Could you check a few things on this model? Use its own coordinates, in mm. Face numbers are marked on the shaded views. A direction names the side the tool comes from. Round coordinates to 2 decimals unless told otherwise and drop trailing zeros. Write each loop counter-clockwise with the first axis right and the second up, starting at its lowest first coordinate (ties: lowest second). Pieces come first, ordered by that corner, then holes. Notation, with made-up numbers: M 14.5,61 L 61.5,61 A24 cw 61.5,99 Z; hole C -28,34.5 d10. An arc over 180 degrees is marked long. One line per item, written item: value. Start each with the question number.
(1) Which directions (+Z, -Z, +X, -X, +Y, -Y) give clear straight access to the entire face, cutting with the end or side of a thin tool? Please do the marked faces 1, 2, 3, 4 and 5.
(2) I want a section at C-C on y = 114. Please give me the cut outline in (x, z), and give its area (3 significant figures).
(3) I want a section at D-D on z = 25. Please give me the cut outline in (x, y).
(4) I'm going to push flat-ended pins straight in: pin 1 Ø4.5 at (x, z) = (-73.15, 20) entering from -Y; pin 2 Ø0.8 at (y, z) = (18.5, 0.5) entering from +X; pin 3 Ø0.6 at (y, z) = (1, 38.5) entering from +X. Where does each tip first touch, or does it pass through?
(5) I want a section at B-B on z = 12. Please give me the cut outline in (x, y).
(6) I want a section at A-A on x = 0. Please give me the cut outline in (y, z).
(7) If I drill on L1, parallel to X at y = 38.5, z = 25; L2, parallel to Y at x = -77.5, z = 30.5; L3, parallel to X at y = 91, z = 19, over which ranges is the centre line in solid material (lowest first)?
(8) Thinking about a two-plate mould opening in X: for the marked faces 6, 7, 8 and 9, which applies, released by +X, released by -X, zero draft, split by the parting line, or undercut?
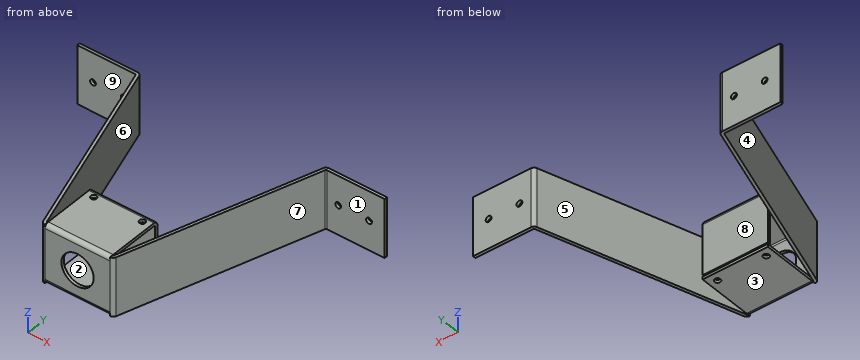
```python
from build123d import *

# Parameters (mm, degrees)
BASE_FLANGE1_DEPTH           = 40
EDGE_FLANGE1_STRIP_W         = 9.4732
EDGE_FLANGE1_STRIP_H         = 2
EDGE_FLANGE1_STRIP_CUT_DEPTH = 44.47497737
EDGE_FLANGE1_DEPTH           = 44.47497737
EDGE_FLANGE2_STRIP_W         = 9.4732
EDGE_FLANGE2_STRIP_H         = 2
EDGE_FLANGE2_STRIP_CUT_DEPTH = 44.47497737
EDGE_FLANGE2_DEPTH           = 44.47497737
EDGE_FLANGE3_STRIP_W         = 9.4732
EDGE_FLANGE3_STRIP_H         = 2
EDGE_FLANGE3_STRIP_CUT_DEPTH = 44.47497737
EDGE_FLANGE3_DEPTH           = 44.47497737
CUT_EXTRUDE1_REACH           = 175.247
SKETCH28_R                   = 11
SKETCH28_R_2                 = 2
SKETCH29_R                   = 2
CUT_EXTRUDE2_DEPTH           = 174.246707232


# Sheet-metal steps are written as plain solids
with BuildPart() as part:
    # Sketch1 → Base-Flange1 (new body)
    with BuildSketch(Plane.XY):
        with BuildLine():
            Line((104.835211483, 130), (65.376911342, 130))
            ThreePointArc((65.376911342, 130), (64.940513549, 129.856810925), (64.67378015, 129.482913293))
            Line((64.67378015, 129.482913293), (24.849746113, 1.921069076))
            ThreePointArc((24.849746113, 1.921069076), (23.858784098, 0.531972879), (22.237488685, 0))
            Line((22.237488685, 0), (-22.237488685, 0))
            ThreePointArc((-22.237488685, 0), (-23.858784098, 0.531972879), (-24.849746113, 1.921069076))
            Line((-24.849746113, 1.921069076), (-64.67378015, 129.482913293))
            ThreePointArc((-64.67378015, 129.482913293), (-64.940513549, 129.856810925), (-65.376911342, 130))
            Line((-65.376911342, 130), (-104.835211483, 130))
            Line((-104.835211483, 130), (-104.835211483, 132))
            Line((-104.835211483, 132), (-65.376911342, 132))
            ThreePointArc((-65.376911342, 132), (-63.755615929, 131.468027121), (-62.764653914, 130.078930924))
            Line((-62.764653914, 130.078930924), (-22.940619877, 2.517086707))
            ThreePointArc((-22.940619877, 2.517086707), (-22.673886478, 2.143189075), (-22.237488685, 2))
            Line((-22.237488685, 2), (22.237488685, 2))
            ThreePointArc((22.237488685, 2), (22.673886478, 2.143189075), (22.940619877, 2.517086707))
            Line((22.940619877, 2.517086707), (62.764653914, 130.078930924))
            ThreePointArc((62.764653914, 130.078930924), (63.755615929, 131.468027121), (65.376911342, 132))
            Line((65.376911342, 132), (104.835211483, 132))
            Line((104.835211483, 132), (104.835211483, 130))
        make_face()
    extrude(amount=BASE_FLANGE1_DEPTH)

    # Edge-Flange1 strip (across the edge) → Edge-Flange1 strip cut (cut)
    with BuildSketch(Plane(origin=(22.237488685, 2, 0), x_dir=(0, 0, 1), z_dir=(-1, 0, 0))):
        with Locations((-2, -1)):
            Rectangle(EDGE_FLANGE1_STRIP_W, EDGE_FLANGE1_STRIP_H)
    extrude(amount=EDGE_FLANGE1_STRIP_CUT_DEPTH, mode=Mode.SUBTRACT)

    # Edge-Flange1 section (across the edge) → Edge-Flange1 (add)
    with BuildSketch(Plane(origin=(22.237488685, 2, 0), x_dir=(0, 0, 1), z_dir=(-1, 0, 0))):
        with BuildLine():
            Line((0, 0.7366), (0, 38))
            Line((0, 38), (2, 38))
            Line((2, 38), (2, 0.7366))
            ThreePointArc((2, 0.7366), (2.215745145, 0.215745145), (2.7366, 0))
            Line((2.7366, 0), (2.7366, -2))
            ThreePointArc((2.7366, -2), (0.801531583, -1.198468417), (0, 0.7366))
        make_face()
    extrude(amount=EDGE_FLANGE1_DEPTH)

    # Edge-Flange2 strip (across the edge) → Edge-Flange2 strip cut (cut)
    with BuildSketch(Plane(origin=(-22.237488685, 2, 40), x_dir=(0, 0, -1), z_dir=(1, 0, 0))):
        with Locations((-2, -1)):
            Rectangle(EDGE_FLANGE2_STRIP_W, EDGE_FLANGE2_STRIP_H)
    extrude(amount=EDGE_FLANGE2_STRIP_CUT_DEPTH, mode=Mode.SUBTRACT)

    # Edge-Flange2 section (across the edge) → Edge-Flange2 (add)
    with BuildSketch(Plane(origin=(-22.237488685, 2, 40), x_dir=(0, 0, -1), z_dir=(1, 0, 0))):
        with BuildLine():
            Line((0, 0.7366), (0, 38))
            Line((0, 38), (2, 38))
            Line((2, 38), (2, 0.7366))
            ThreePointArc((2, 0.7366), (2.215745145, 0.215745145), (2.7366, 0))
            Line((2.7366, 0), (2.7366, -2))
            ThreePointArc((2.7366, -2), (0.801531583, -1.198468417), (0, 0.7366))
        make_face()
    extrude(amount=EDGE_FLANGE2_DEPTH)

    # Edge-Flange3 strip (across the edge) → Edge-Flange3 strip cut (cut)
    with BuildSketch(Plane(origin=(-22.237488685, 40, 38), x_dir=(0, -1, 0), z_dir=(1, 0, 0))):
        with Locations((-2, -1)):
            Rectangle(EDGE_FLANGE3_STRIP_W, EDGE_FLANGE3_STRIP_H)
    extrude(amount=EDGE_FLANGE3_STRIP_CUT_DEPTH, mode=Mode.SUBTRACT)

    # Edge-Flange3 section (across the edge) → Edge-Flange3 (add)
    with BuildSketch(Plane(origin=(-22.237488685, 40, 38), x_dir=(0, -1, 0), z_dir=(1, 0, 0))):
        with BuildLine():
            Line((0, 0.7366), (0, 35))
            Line((0, 35), (2, 35))
            Line((2, 35), (2, 0.7366))
            ThreePointArc((2, 0.7366), (2.215745145, 0.215745145), (2.7366, 0))
            Line((2.7366, 0), (2.7366, -2))
            ThreePointArc((2.7366, -2), (0.801531583, -1.198468417), (0, 0.7366))
        make_face()
    extrude(amount=EDGE_FLANGE3_DEPTH)

    # Sketch28 → Cut-Extrude1 (cut, up to next)
    with BuildSketch(Plane.XZ, mode=Mode.PRIVATE) as cut_extrude1_sk1:
        with Locations(Location((0, 20, 0), (0, 0, 270))):
            Circle(SKETCH28_R)
    cut_extrude1_tool1 = extrude(cut_extrude1_sk1.sketch, amount=-CUT_EXTRUDE1_REACH, mode=Mode.PRIVATE) & part.part
    # Sketch28 → Cut-Extrude1 (cut, up to next)
    with BuildSketch(Plane.XZ, mode=Mode.PRIVATE) as cut_extrude1_sk2:
        with Locations((73.154329826, 20)):
            Circle(SKETCH28_R_2)
    cut_extrude1_tool2 = extrude(cut_extrude1_sk2.sketch, amount=-CUT_EXTRUDE1_REACH, mode=Mode.PRIVATE) & part.part
    # Sketch28 → Cut-Extrude1 (cut, up to next)
    with BuildSketch(Plane.XZ, mode=Mode.PRIVATE) as cut_extrude1_sk3:
        with Locations((94.167570852, 20)):
            Circle(SKETCH28_R_2)
    cut_extrude1_tool3 = extrude(cut_extrude1_sk3.sketch, amount=-CUT_EXTRUDE1_REACH, mode=Mode.PRIVATE) & part.part
    # Sketch28 → Cut-Extrude1 (cut, up to next)
    with BuildSketch(Plane.XZ, mode=Mode.PRIVATE) as cut_extrude1_sk4:
        with Locations((-94.167570852, 20)):
            Circle(SKETCH28_R_2)
    cut_extrude1_tool4 = extrude(cut_extrude1_sk4.sketch, amount=-CUT_EXTRUDE1_REACH, mode=Mode.PRIVATE) & part.part
    # Sketch28 → Cut-Extrude1 (cut, up to next)
    with BuildSketch(Plane.XZ, mode=Mode.PRIVATE) as cut_extrude1_sk5:
        with Locations((-73.154329826, 20)):
            Circle(SKETCH28_R_2)
    cut_extrude1_tool5 = extrude(cut_extrude1_sk5.sketch, amount=-CUT_EXTRUDE1_REACH, mode=Mode.PRIVATE) & part.part
    add(cut_extrude1_tool1.solids().sort_by_distance((0, 0, 20))[0], mode=Mode.SUBTRACT)
    add(cut_extrude1_tool2.solids().sort_by_distance((73.15433, 0, 20))[0], mode=Mode.SUBTRACT)
    add(cut_extrude1_tool3.solids().sort_by_distance((94.167571, 0, 20))[0], mode=Mode.SUBTRACT)
    add(cut_extrude1_tool4.solids().sort_by_distance((-94.167571, 0, 20))[0], mode=Mode.SUBTRACT)
    add(cut_extrude1_tool5.solids().sort_by_distance((-73.15433, 0, 20))[0], mode=Mode.SUBTRACT)

    # Sketch29 → Cut-Extrude2 (cut, through all)
    with BuildSketch(Plane(origin=(0, 0, 0), x_dir=(-1, 0, 0), z_dir=(0, 0, -1))):
        with Locations(Location((-16.618744342, 34.381255658, 0), (0, 0, 90))):
            Circle(SKETCH29_R)
        with Locations(Location((16.618744342, 34.381255658, 0), (0, 0, 90))):
            Circle(SKETCH29_R)
    extrude(amount=-CUT_EXTRUDE2_DEPTH, mode=Mode.SUBTRACT)


solid = part.part
```
Found:
1. face 1: +Z, -Z, +X, -Y
1. face 2: +Y
1. face 3: -Z, +X, -X, +Y, -Y
1. face 4: +Z, -Z, -X, -Y
1. face 5: +Z, -Z, +Y
2. outline: M -59.84,0 L -57.74,0 L -57.74,40 L -59.84,40 Z; M 57.74,0 L 59.84,0 L 59.84,40 L 57.74,40 Z
2. area: 168 mm²
3. outline: M -104.84,130 L -65.38,130 A0.74 cw -64.67,129.48 L -24.85,1.92 A2.74 ccw -22.24,0 L -9.8,0 L -9.8,2 L -22.24,2 A0.74 cw -22.94,2.52 L -62.76,130.08 A2.74 ccw -65.38,132 L -104.84,132 Z; M -22.24,38 L 22.24,38 L 22.24,40 L -22.24,40 Z; M 9.8,0 L 22.24,0 A2.74 ccw 24.85,1.92 L 64.67,129.48 A0.74 cw 65.38,130 L 104.84,130 L 104.84,132 L 65.38,132 A2.74 ccw 62.76,130.08 L 22.94,2.52 A0.74 cw 22.24,2 L 9.8,2 Z
4. pin 1: stops at y = 130
4. pin 2: stops at x = 30.15
4. pin 3: stops at x = 24.57
5. outline: M -104.84,130 L -65.38,130 A0.74 cw -64.67,129.48 L -24.85,1.92 A2.74 ccw -22.24,0 L -7.55,0 L -7.55,2 L -22.24,2 A0.74 cw -22.94,2.52 L -62.76,130.08 A2.74 ccw -65.38,132 L -104.84,132 Z; M -22.24,38 L 22.24,38 L 22.24,40 L -22.24,40 Z; M 7.55,0 L 22.24,0 A2.74 ccw 24.85,1.92 L 64.67,129.48 A0.74 cw 65.38,130 L 104.84,130 L 104.84,132 L 65.38,132 A2.74 ccw 62.76,130.08 L 22.94,2.52 A0.74 cw 22.24,2 L 7.55,2 Z
6. outline: M 0,2.74 A2.74 ccw 2.74,0 L 40,0 L 40,2 L 2.74,2 A0.74 cw 2,2.74 L 2,9 L 0,9 Z; M 0,31 L 2,31 L 2,37.26 A0.74 cw 2.74,38 L 37.26,38 A0.74 cw 38,37.26 L 38,3 L 40,3 L 40,37.26 A2.74 ccw 37.26,40 L 2.74,40 A2.74 ccw 0,37.26 Z
7. L1: x = -36.27 to -34.17, -22.24 to 22.24, 34.17 to 36.27
7. L2: y = 130 to 132
7. L3: x = -52.66 to -50.56, 50.56 to 52.66
8. face 6: undercut
8. face 7: released by +X
8. face 8: undercut
8. face 9: zero draft
